The listing builds one solid part. Answer for the finished solid, in the listing's coordinates (mm). A direction names the side the tool comes from. Coordinates: 2 decimals unless noted, no trailing zeros. Order: outer loops, then holes, each group sorted by start corner. A loop starts at its lowest first (then second) coordinate and runs counter-clockwise, first axis right, second up.
Autodesk Inventor part; units mm, degrees
ref_plane "YZ Plane" through (0, 0, 0) normal (1, 0, 0) x (0, 1, 0)
ref_plane "XZ Plane" through (0, 0, 0) normal (0, 1, 0) x (-1, 0, 0)
ref_plane "XY Plane" through (0, 0, 0) normal (0, 0, 1) x (1, 0, 0)
sketch "Esboço1" plane through (0, 0, 0) normal (1, 0, 0) x (0, 1, 0)
  line L0 (0.3875, 55) -> (-38.7875, 55)
  line L1 (-38.7875, 55) -> (-38.7875, -55)
  line L2 (-38.7875, -55) -> (38.7875, -55)
  line L3 (38.7875, -55) -> (0.3875, 55)
  point P0 (0, 0)
  point P1 (19.5875, 0)
  point P2 (0, -55)
  dimension "d4" = 77.575
  dimension "d5" = 110
  dimension "d6" = 39.175
extrude "Extrusão1" add sketch "Esboço1" along normal blind 4
sketch "Esboço2" plane through (0, -38.7875, -55) normal (0, 0, -1) x (-1, 0, 0)
  line L0 (0, 0) -> (-4, 0)
  line L1 (0, 77.575) -> (-4, 77.575)
  line L2 (-4, 0) -> (-4, 77.575)
  line L3 (0, 39.175) -> (0, 0)
  line L4 (-4, 51.2875) -> (0, 51.2875)
  line L5 (0, 51.2875) -> (0, 26.2875)
  line L6 (0, 26.2875) -> (-4, 26.2875)
  line L7 (-4, 26.2875) -> (-4, 51.2875)
  point P0 (0, 38.7875)
  dimension "d7" = 77.575
  dimension "d8" = 25
  dimension "d9" = 26.2875
extrude "Extrusão2" add sketch "Esboço2" along normal blind 4 contours L6 L2 L4 L5 L3
properties part number "suporte"
(1) This flat-tipped pin is pushed along its axis until it touches: pin 1 Ø2 at (x, y) = (1, -24) entering from -Z. Where does it stop, or does it pass through?
(2) Find section C-C (z = 44.5). Write down the section's boundary in (x, y).
(3) Find section A-A (x = 0.6). Write down the section's boundary in (y, z), and give its area (3 significant figures).
(4) For faces 1 (the face through (2, 0, -59)), 2 (the face through (2, -26, -55)), 3 (the face through (2, 12.5, -57)), determine the directions among +Z, -Z, +X, -X, +Y, -Y from which every point of the face is accessible in a straight line to the end or side of a thin tool.
(5) Find section B-B (y = -32.5). Write down the section's boundary in (x, z).
(6) Consider line 1 (Z direction, x = 0.7, y = -22); line 2 (Y direction, x = 2.35, z = -12.5); line 3 (Y direction, x = 3.7, z = 0.5). Determine where each line is inside the solid, lowest interval first.
Findings below:
1. pin 1: stops at z = -55
2. outline: (0, -38.79) - (4, -38.79) - (4, 4.05) - (0, 4.05) - close
3. outline: (-38.79, -55) - (-12.5, -55) - (-12.5, -59) - (12.5, -59) - (12.5, -55) - (38.79, -55) - (0.39, 55) - (-38.79, 55) - close
3. area: 6,520 mm2
4. face 1: -Z, +X, -X, +Y, -Y
4. face 2: -Z, +X, -X, -Y
4. face 3: -Z, +X, -X, +Y
5. outline: (0, -55) - (4, -55) - (4, 55) - (0, 55) - close
6. line 1: z = -55 to 55
6. line 2: y = -38.79 to 23.95
6. line 3: y = -38.79 to 19.41
